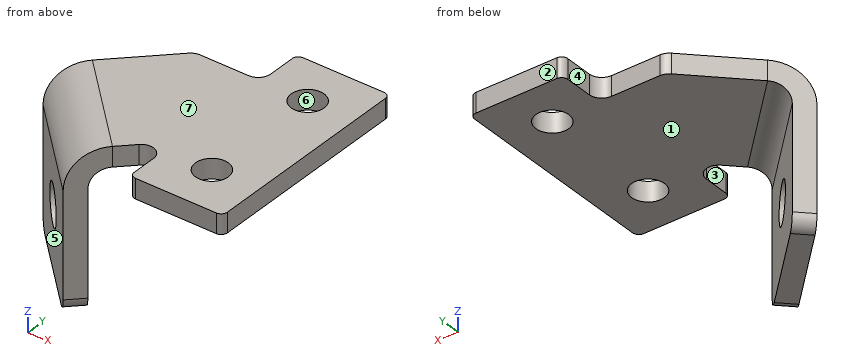
Autodesk Inventor part; units mm, degrees
ref_plane "YZ Plane" through (0, 0, 0) normal (1, 0, 0) x (0, 1, 0)
ref_plane "XZ Plane" through (0, 0, 0) normal (0, 1, 0) x (-1, 0, 0)
ref_plane "XY Plane" through (0, 0, 0) normal (0, 0, 1) x (1, 0, 0)
sketch "Sketch1" plane through (0, 0, 0) normal (0, 0, 1) x (1, 0, 0)
  line L0 (0, -21.2132) -> (-21.2132, 0) construction
  line L1 (-21.2132, 0) -> (0, 21.2132) construction
  line L2 (0, 21.2132) -> (21.2132, 0) construction
  line L3 (21.2132, 0) -> (0, -21.2132) construction
  line L4 (0, -21.2132) -> (0, 21.2132) construction
  line L5 (-21.2132, 0) -> (21.2132, 0) construction
  line L6 (43, 4) -> (28, 4)
  line L7 (28, 4) -> (28, 39)
  line L8 (28, 39) -> (43, 39)
  line L9 (43, 39) -> (43, 4)
  line L10 (43, 4) -> (28, 39) construction
  line L11 (28, 4) -> (43, 39) construction
  line L12 (35.5, 11.5) -> (35.5, 31.5) construction
  line L13 (17.6777, 3.5355) -> (3.5355, 17.6777)
  line L14 (3.5355, 17.6777) -> (17.3579, 31.5)
  line L15 (17.3579, 31.5) -> (28, 31.5)
  line L16 (17.6777, 3.5355) -> (25.6421, 11.5)
  line L17 (25.6421, 11.5) -> (28, 11.5)
  line L18 (28, 11.5) -> (28, 31.5)
  point P0 (0, 0)
  point P1 (35.5, 21.5)
  point P2 (0, 0)
  point P3 (0, 0)
  point P4 (35.5, 21.5)
  point P5 (43, 21.5)
  point P6 (10.6066, 10.6066)
  point P7 (28, 21.5)
  dimension "d0" = 30
  dimension "d1" = 28
  dimension "d2" = 21.5
  dimension "d3" = 35
  dimension "d5" = 20
  dimension "d6" = 7.5
  dimension "d7" = 7.5
  dimension "d8" = 7.5
  dimension "d11" = 20
  dimension "d12" = 20
extrude "Plate2" add sketch "Sketch1" against normal blind 3.175
sketch "Sketch2" plane through (5.7806, 19.9227, 0) normal (-0.7071068, -0.7071068, 0) x (0.7071068, -0.7071068, 0)
  line L0 (20, 0) -> (0, 0)
  line L1 (0, 0) -> (0, -25)
  line L2 (0, -25) -> (20, -25)
  line L3 (20, -25) -> (20, 0)
edge flange "Flange1" height 25 angle 90 thickness 3.175 bend radius 3.175 thickness toward (-0.7071068, -0.7071068, 0) relief tear relief width 3.175 relief depth 1.5875 edges at (10.6066, 10.6066, -3.175) wall of the first edge with corners at (19.9227, 5.7806, 0) (5.7806, 19.9227, 0) (5.7806, 19.9227, -25) (19.9227, 5.7806, -25)
bend "Bend1"
corner "Corner1"
fillet "Fillet1" radius 2 4 edges at (25.6421, 11.5, -1.5875) (28, 11.5, -1.5875) (28, 31.5, -1.5875) (17.3579, 31.5, -1.5875)
sketch "Sketch3" plane through (3.5355, 17.6777, -6.35) normal (-0.7071068, -0.7071068, 0) x (-0.7071068, 0.7071068, 0)
  line L0 (0, -1.35) -> (-20, -1.35) construction
  line L1 (-20, -1.35) -> (-20, 18.65) construction
  line L2 (-20, 18.65) -> (0, 18.65) construction
  line L3 (0, 18.65) -> (0, -1.35) construction
  line L4 (0, -1.35) -> (-20, 18.65) construction
  line L5 (-20, -1.35) -> (0, 18.65) construction
  point P0 (-10, -6.35)
  point P1 (-10, 8.65)
hole "Hole2" at (10.6066, 10.6066, -15) direction (0.7071068, 0.7071068, 0) diameter 6.3 end through all
fillet "Fillet2" radius 2 2 edges at (4.6581, 18.8002, -25) (18.8002, 4.6581, -25)
fillet "Fillet3" radius 1 4 edges at (28, 4, -1.5875) (28, 39, -1.5875) (43, 4, -1.5875) (43, 39, -1.5875)
hole "Hole1" at (35.5, 31.5, 0) at (35.5, 11.5, 0) direction (0, 0, -1) diameter 5.3 end through all
equation "\"d6\" = d7"
equation "\"d8\" = d6"
equation "\"d12\" = d11"
equation "\"d32\" = Thickness"
equation "\"d13\" = Thickness"
equation "\"d14\" = BendReliefWidth"
equation "\"d15\" = BendReliefDepth"
equation "\"d16\" = MinimumRemnant"
equation "\"d17\" = TransitionRadius"
equation "\"d20\" = BendRadius"
equation "\"d21\" = CornerReliefSize"
equation "\"d22\" = GapSize"
equation "\"d23\" = JacobiRadiusSize"
equation "\"BendReliefWidth\" = Thickness"
equation "\"BendReliefDepth\" = 0.5 * Thickness"
equation "\"CornerReliefSize\" = 4 * Thickness"
equation "\"MinimumRemnant\" = 2 * Thickness"
equation "\"TransitionRadius\" = BendRadius"
equation "\"JacobiRadiusSize\" = BendRadius"
equation "\"GapSize\" = Thickness"
properties part number "External Frame Corner Bracket" material "Aluminum 6061"
Design review of the part built by this model. Coordinates are the model's own, in mm. Face numbers are marked on the shaded views. A direction names the side the tool comes from. Coordinates: 2 decimals unless noted, no trailing zeros. Order: outer loops, then holes, each group sorted by start corner. A loop starts at its lowest first (then second) coordinate and runs counter-clockwise, first axis right, second up. Notation, with made-up numbers: (-40, 22) -> (-16, 22) arc R25 cw to (-16, 40) -> close; hole circle Ø6 at (33.5, 30.5). An arc over 180 degrees is marked (long way). One line per item, written item: value. Start each with the question number.
Q1. Tool access review of the marked faces 1, 2, 3 and 4: name each direction out of +Z, -Z, +X, -X, +Y, -Y from which nothing blocks a thin tool from reaching the whole face with its end or side.
Q2. Mouldability with a two-part tool opening along Y and no side actions: class the marked faces 5, 6 and 7 as pulls with the +Y half, pulls with the -Y half, needs draft (parallel to the pull), parting line crosses it, or undercut.
Q3. Take a section at C-C, the plane y = 11.5. Give the number of separate pieces and of enclosed holes in the cut face, then the cut area to 3 significant figures.
Q4. Insertion check: pin 1 Ø17.5 at (x, y) = (18.5, 17.5) entering from -Z; pin 2 Ø8 at (x, z) = (11.5, -4.5) entering from -Y; pin 3 Ø1 at (x, z) = (21.5, -1) entering from +Y; pin 4 Ø1 at (y, z) = (8, -12) entering from +X. Each pin has a flat end and moves straight along its axis. Give the tip position at first contact, or say it passes through.
Q5. Take a section at B-B, the plane z = -16. State the section outline as (x, y) points.
Q6. For probe 1 along Y at (x, z) = (35.5, -0.7); probe 2 along Y at (x, z) = (30, -2); probe 3 along Z at (x, y) = (26, 26) (3 decimals), list the stretches that pass through material, from the lowest coordinate up.
Q7. Take a section at D-D, the plane z = -21.25. State the section outline as (x, y) points, then the cut area to 3 significant figures.
Q8. Take a section at A-A, the plane x = 33.5. State the section outline as (y, z) points (3 decimals), then the cut area to 3 significant figures.
Values follow:
1. face 1: -Z, +X, +Y
1. face 2: +Z, -Z, +X, -X, +Y
1. face 3: +Z, -Z, -Y
1. face 4: +Z, -Z, -X, +Y
2. face 5: pulls with the -Y half
2. face 6: undercut
2. face 7: needs draft
3. separate pieces: 3
3. enclosed holes: 0
3. area: 151 mm2
4. pin 1: stops at z = -25
4. pin 2: stops at y = 5.92
4. pin 3: stops at y = 31.5
4. pin 4: stops at x = 18.2
5. outline: (3.54, 17.68) -> (8.49, 12.72) -> (10.74, 14.96) -> (5.78, 19.92) -> close; (12.72, 8.49) -> (17.68, 3.54) -> (19.92, 5.78) -> (14.96, 10.74) -> close
6. probe 1: y = 4 to 8.85, 14.15 to 28.85, 34.15 to 39
6. probe 2: y = 4 to 39
6. probe 3: z = -3.175 to 0
7. outline: (3.54, 17.68) -> (17.68, 3.54) -> (19.92, 5.78) -> (5.78, 19.92) -> close
7. area: 63.5 mm2
8. outline: (4, -3.175) -> (9.761, -3.175) -> (9.761, 0) -> (4, 0) -> close; (13.239, -3.175) -> (29.761, -3.175) -> (29.761, 0) -> (13.239, 0) -> close; (33.239, -3.175) -> (39, -3.175) -> (39, 0) -> (33.239, 0) -> close
8. area: 89.0 mm2
